```python
from build123d import *

# Parameters (mm, degrees)
SKETCH_R        = 4.5
PAD_DEPTH       = 6
CHAMFER_SIZE    = 0.5
CHAMFER001_SIZE = 0.5


with BuildPart() as part:
    # Sketch → Pad (new body)
    with BuildSketch(Plane.XY):
        Polygon((4.907477, 8.5), (-4.907477, 8.5), (-9.814955, 0), (-4.907477, -8.5), (4.907477, -8.5), (9.814955, 0), align=None)
        Circle(SKETCH_R, mode=Mode.SUBTRACT)
    extrude(amount=PAD_DEPTH)

    # Chamfer
    chamfer_edges = [part.edges().sort_by_distance(p)[0] for p in [
        (0, -8.5, 6),
        (-7.361216, -4.25, 6),
        (-7.361216, 4.25, 6),
        (0, 8.5, 6),
        (7.361216, 4.25, 6),
        (7.361216, -4.25, 6),
    ]]
    chamfer(chamfer_edges, length=CHAMFER_SIZE)

    # Chamfer001
    chamfer001_edges = [part.edges().sort_by_distance(p)[0] for p in [
        (7.361216, -4.25, 0),
        (0, -8.5, 0),
        (-7.361216, -4.25, 0),
        (-7.361216, 4.25, 0),
        (0, 8.5, 0),
        (7.361216, 4.25, 0),
    ]]
    chamfer(chamfer001_edges, length=CHAMFER001_SIZE)


solid = part.part
```
Work out the finished part from the listing and answer in its coordinate system (mm). Give positions to 0.01 mm unless a question says otherwise; leave off trailing zeros. Loops run counter-clockwise (first coordinate to the right, second up) from the corner with the lowest first, then second, coordinate; pieces in that order, holes last. Notation, with made-up numbers: (70.25, 31) - (120.25, 31) arc R20 cw to (120.25, 70) - close; hole circle Ø4 at (26, 55). An arc over 180 degrees is marked (long way). Use CSV: the item, a comma, the result in double quotes. Start each with the question number.
(1) Find section A-A, the plane x = 0. Determine the outline of the cut face in (y, z), plus the area to 3 significant figures.
(2) This flat-tipped pin is pushed along its axis until it touches: pin 1 (1 mm diameter, centred on y = 6.5, z = 2.5, fed in from -X). Where does it stop, or does it pass through?
(3) Determine the mould class of faces 1 (the face through (-7.327, 4.31, 2.965)), 2 (the face through (7.18, 4.06, 0.25)), 3 (the face through (0, -8.5, 3)), 4 (the face through (-0.59, 4.46, 2.96)) for opening direction X: released by +X, released by -X, zero draft, split by the parting line, or undercut.
(4) Find section C-C, the plane y = 0.5. Determine the outline of the cut face in (x, z), plus the area to 3 significant figures.
(5) Find the intervals of material crossed by L1, parallel to Y at x = 0, z = 3.1; L2, parallel to X at y = 1.75, z = 3.25; L3, parallel to Y at x = -2.5, z = 0.75, in increasing order.
(6) Find section D-D, the plane x = 7.5. Determine the outline of the cut face in (y, z).
(7) Find section B-B, the plane z = 4.5. Determine the outline of the cut face in (x, y), plus the area to 3 significant figures.
Results found:
1,outline,"(-8.5, 0.5) - (-8, 0) - (-4.5, 0) - (-4.5, 6) - (-8, 6) - (-8.5, 5.5) - close; (4.5, 0) - (8, 0) - (8.5, 0.5) - (8.5, 5.5) - (8, 6) - (4.5, 6) - close"
1,area,"47.5 mm^2"
2,pin 1,"x = -6.35"
3,face 1,"released by -X"
3,face 2,"released by +X"
3,face 3,"zero draft"
3,face 4,"undercut"
4,outline,"(-9.53, 0.5) - (-8.95, 0) - (-4.47, 0) - (-4.47, 6) - (-8.95, 6) - (-9.53, 5.5) - close; (4.47, 0) - (8.95, 0) - (9.53, 0.5) - (9.53, 5.5) - (8.95, 6) - (4.47, 6) - close"
4,area,"60.1 mm^2"
5,L1,"-8.5 to -4.5, 4.5 to 8.5"
5,L2,"-8.8 to -4.15, 4.15 to 8.8"
5,L3,"-8.5 to -3.74, 3.74 to 8.5"
6,outline,"(-4.01, 0.5) - (-3.01, 0) - (3.01, 0) - (4.01, 0.5) - (4.01, 5.5) - (3.01, 6) - (-3.01, 6) - (-4.01, 5.5) - close"
7,outline,"(-9.81, 0) - (-4.91, -8.5) - (4.91, -8.5) - (9.81, 0) - (4.91, 8.5) - (-4.91, 8.5) - close; hole circle Ø9 at (0, 0)"
7,area,"187 mm^2"
